Part model, mm, in its own coordinate system. Round coordinates to 2 decimals unless told otherwise and drop trailing zeros. Order: outer loops, then holes, each group sorted by start corner. A loop starts at its lowest first (then second) coordinate and runs counter-clockwise, first axis right, second up. Notation, with made-up numbers: M 19,77 L 24,77 A23 cw 24,100 Z; hole C 56,-2 d2. An arc over 180 degrees is marked long. One line per question, with ' | ' between items.
from build123d import *

# Parameters (mm, degrees)
F1_DEPTH = 3
F2_W     = 10
F2_H     = 5.5
F3_DEPTH = 25
F4_R     = 12.75
F5_DEPTH = 25


with BuildPart() as f1:
    # F0 (on Right) → F1 (new body)
    with BuildSketch(Plane.YZ):
        Polygon((80, 30), (0, 30), (-80, 30), (-80, -30), (0, -30), (80, -30), align=None)
    extrude(amount=F1_DEPTH)

    # F2 (on face) → F3 (cut)
    with BuildSketch(Plane.YZ.offset(3)):
        with Locations((-55, -4.25)):
            Rectangle(F2_W, F2_H)
        with Locations((-55, 4.25)):
            Rectangle(F2_W, F2_H)
        with Locations((55, 4.25)):
            Rectangle(F2_W, F2_H)
        with Locations((55, -4.25)):
            Rectangle(F2_W, F2_H)
    extrude(amount=-F3_DEPTH, mode=Mode.SUBTRACT)

    # F4 (on face) → F5 (cut)
    with BuildSketch(Plane.YZ.offset(3)):
        Circle(F4_R)
    extrude(amount=-F5_DEPTH, mode=Mode.SUBTRACT)


solid = f1.part
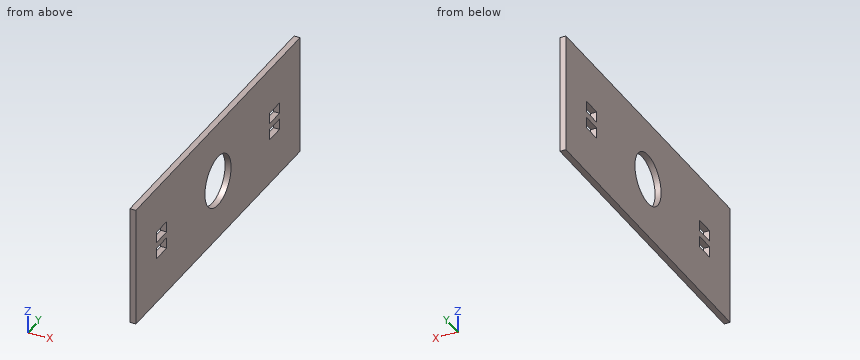
1) Saw through at B-B (z = 0). List the corners of the cut face in (x, y), plus the area to 4 significant figures.
The answers:
outline: M 0,-80 L 3,-80 L 3,-12.75 L 0,-12.75 Z; M 0,12.75 L 3,12.75 L 3,80 L 0,80 Z | area: 403.5 mm²
2) Saw through at C-C (x = 1.8). List the corners of the cut face in (y, z), plus the area to 3 significant figures.
The answers:
outline: M -80,-30 L 80,-30 L 80,30 L -80,30 Z; hole M -60,-7 L -50,-7 L -50,-1.5 L -60,-1.5 Z; hole M -60,1.5 L -50,1.5 L -50,7 L -60,7 Z; hole C 0,0 d25.5; hole M 50,-7 L 60,-7 L 60,-1.5 L 50,-1.5 Z; hole M 50,1.5 L 60,1.5 L 60,7 L 50,7 Z | area: 8,870 mm²
3) Probe line 1 (Z direction, x = 2.4, y = -55); line 2 (Z direction, x = 1.25, y = 0); line 3 (Y direction, x = 1.95, z = -3). List the from-to ranges inside material, lowest first. Write a range as [from, to].
The answers:
line 1: z = [-30, -7], [-1.5, 1.5], [7, 30] | line 2: z = [-30, -12.75], [12.75, 30] | line 3: y = [-80, -60], [-50, -12.39], [12.39, 50], [60, 80]
4) Saw through at D-D (y = 0). List the corners of the cut face in (x, z), plus the area to 4 significant figures.
The answers:
outline: M 0,-30 L 3,-30 L 3,-12.75 L 0,-12.75 Z; M 0,12.75 L 3,12.75 L 3,30 L 0,30 Z | area: 103.5 mm²
5) Saw through at A-A (y = 53). List the corners of the cut face in (x, z).
The answers:
outline: M 0,-30 L 3,-30 L 3,-7 L 0,-7 Z; M 0,-1.5 L 3,-1.5 L 3,1.5 L 0,1.5 Z; M 0,7 L 3,7 L 3,30 L 0,30 Z
